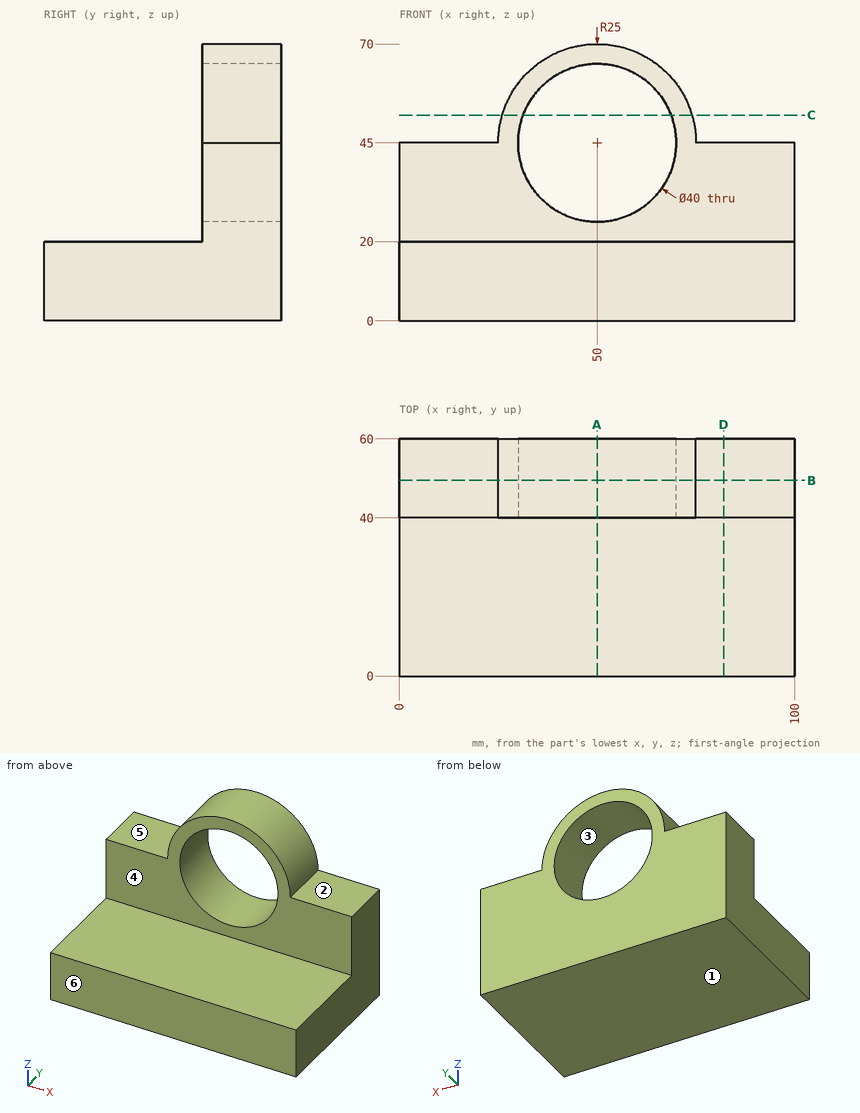
For this review, use the dimensioned drawing (mm, ordinates from the lowest corner) and the shaded views. A direction names the side the tool comes from. Give positions to 0.01 mm unless a question says otherwise; leave off trailing zeros. Order: outer loops, then holes, each group sorted by start corner. A loop starts at its lowest first (then second) coordinate and runs counter-clockwise, first axis right, second up.
1. Add section D-D, the plane x = 82. State the section outline as (y, z) points.
Solution:
outline: (0, 0) - (60, 0) - (60, 45) - (40, 45) - (40, 20) - (0, 20) - close
2. For pin 1 Ø10 at (x, y) = (33.5, 47) entering from +Z; pin 2 Ø10 at (y, z) = (13.5, 10) entering from -X; pin 3 Ø8 at (x, y) = (61, 50.5) entering from +Z; pin 4 Ø12 at (x, y) = (29, 15.5) entering from +Z, all flat-tipped, find the tip position at first contact; note any pin that passes through.
Solution:
pin 1: stops at z = 67.2
pin 2: stops at x = 0
pin 3: stops at z = 69
pin 4: stops at z = 20
3. To check wall thickness, follow L1, parallel to Z at x = 50, y = 53; L2, parallel to Z at x = 77.5, y = 46; L3, parallel to Y at x = 57.5, z = 65.5. State the ranges of each line that lie inside material, in increasing order.
Solution:
L1: z = 0 to 25, 65 to 70
L2: z = 0 to 45
L3: y = 40 to 60
4. Tool access review of the marked faces 4, 5 and 6: name each direction out of +Z, -Z, +X, -X, +Y, -Y from which nothing blocks a thin tool from reaching the whole face with its end or side.
Solution:
face 4: +Z, +X, -X, -Y
face 5: +Z, -X, +Y, -Y
face 6: +Z, -Z, +X, -X, -Y
5. Add section C-C, the plane z = 52. State the section outline as (x, y) points (3 decimals).
Solution:
outline: (26, 40) - (31.265, 40) - (31.265, 60) - (26, 60) - close; (68.735, 40) - (74, 40) - (74, 60) - (68.735, 60) - close
6. Mouldability with a two-part tool opening along Z and no side actions: class the marked faces 1, 2 and 3 as +Z half, -Z half, draft (parallel to the pull), parting line (faces both ways), or undercut.
Solution:
face 1: -Z half
face 2: +Z half
face 3: undercut
7. Add section A-A, the plane x = 50. State the section outline as (y, z) points, then the cut area to 3 significant figures.
Solution:
outline: (0, 0) - (60, 0) - (60, 25) - (40, 25) - (40, 20) - (0, 20) - close; (40, 65) - (60, 65) - (60, 70) - (40, 70) - close
area: 1,400 mm2
8. Add section B-B, the plane y = 49.5. State the section outline as (x, z) points.
Solution:
outline: (0, 0) - (100, 0) - (100, 45) - (75, 45) arc R25 ccw to (25, 45) - (0, 45) - close; hole circle Ø40 at (50, 45)
